```python
from build123d import *

# Parameters (mm, degrees)
SKETCH1_W                           = 558.8
SKETCH1_H                           = 50.8
BOSS_EXTRUDE1_DEPTH                 = 12.7
SKETCH2_W                           = 19.05
SKETCH2_H                           = 44.45
CUT_EXTRUDE1_DEPTH                  = 560.521125607
F_1_4_20_TAPPED_HOLE1_D             = 5.1054
F_10_32_TAPPED_HOLE1_D              = 4.0386
F_10_32_TAPPED_HOLE1_DEPTH          = 5.08
F_10_32_TAPPED_HOLE1_TIP            = 1.213317848
F_5_32_0_15625_DIAMETER_HOLE1_D     = 3.96875
F_5_32_0_15625_DIAMETER_HOLE1_DEPTH = 5.08
F_5_32_0_15625_DIAMETER_HOLE1_TIP   = 1.192332791


with BuildPart() as part:
    # Sketch1 → Boss-Extrude1 (new, symmetric)
    with BuildSketch(Plane.XY):
        Rectangle(SKETCH1_W, SKETCH1_H)
    extrude(amount=BOSS_EXTRUDE1_DEPTH, both=True)

    # Sketch2 → Cut-Extrude1 (cut, through all)
    with BuildSketch(Plane(origin=(279.4, 0, 0), x_dir=(0, 0, -1), z_dir=(1, 0, 0))):
        Rectangle(SKETCH2_W, SKETCH2_H)
    extrude(amount=-CUT_EXTRUDE1_DEPTH, mode=Mode.SUBTRACT)

    # 1/4-20 Tapped Hole1 (through all)
    with Locations(Plane.XY.offset(12.7)):
        with Locations((-260.35, 12.7), (-260.35, -12.7), (260.35, 12.7), (260.35, -12.7)):
            Hole(F_1_4_20_TAPPED_HOLE1_D / 2)

    # #10-32 Tapped Hole1
    with Locations(Plane(origin=(0, 0, -12.7), x_dir=(-1, 0, 0), z_dir=(0, 0, -1))):
        with Locations((-190.5, -13.49375), (-114.3, -13.49375), (-38.1, -13.49375), (38.1, -13.49375), (114.3, -13.49375), (190.5, -13.49375)):
            Hole(F_10_32_TAPPED_HOLE1_D / 2, depth=F_10_32_TAPPED_HOLE1_DEPTH)
            with Locations((0, 0, -(F_10_32_TAPPED_HOLE1_DEPTH + F_10_32_TAPPED_HOLE1_TIP / 2))):  # 118° drill point
                Cone(0, F_10_32_TAPPED_HOLE1_D / 2, F_10_32_TAPPED_HOLE1_TIP, mode=Mode.SUBTRACT)

    # 5/32 (0.15625) Diameter Hole1
    with Locations(Plane(origin=(0, 25.4, 0), x_dir=(1, 0, 0), z_dir=(0, 1, 0))):
        with Locations((-34.925, 0), (34.925, 0)):
            Hole(F_5_32_0_15625_DIAMETER_HOLE1_D / 2, depth=F_5_32_0_15625_DIAMETER_HOLE1_DEPTH)
            with Locations((0, 0, -(F_5_32_0_15625_DIAMETER_HOLE1_DEPTH + F_5_32_0_15625_DIAMETER_HOLE1_TIP / 2))):  # 118° drill point
                Cone(0, F_5_32_0_15625_DIAMETER_HOLE1_D / 2, F_5_32_0_15625_DIAMETER_HOLE1_TIP, mode=Mode.SUBTRACT)


solid = part.part
```
Check sheet for the modelled part. Datum: model origin and axes. Units: mm. A direction names the side the tool comes from. Round coordinates to 2 decimals unless told otherwise and drop trailing zeros. Loops run counter-clockwise (first coordinate to the right, second up) from the corner with the lowest first, then second, coordinate; pieces in that order, holes last. Notation, with made-up numbers: (21.5, 54.5) -> (64.5, 54.5) arc R22 ccw to (64.5, 81.5) -> close; hole circle Ø3 at (75, 8). An arc over 180 degrees is marked (long way). Write item = value, one per line. Start each with the question number.
1) Sectioned sample at B-B, the plane y = -4.5. Record the cut outline in (x, z) (3 decimals), plus the area to 3 significant figures.
2) Thickness scan on probe 1 along Y at (x, z) = (260.35, -11.8); probe 2 along X at (y, z) = (-12, 10.75); probe 3 along Z at (x, y) = (-226, -12) (3 decimals). Record the ranges inside material, lowest first.
3) Gauge pin test, flat ends, axial feed: pin 1 Ø2.5 at (x, y) = (114.3, -13.49) entering from -Z (3 decimals); pin 2 Ø4 at (x, y) = (260.35, 12.7) entering from -Z. Record the tip position at first contact, or that the pin passes through.
4) Sectioned sample at A-A, the plane x = 76.5. Record the cut outline in (y, z) (3 decimals).
5) Release check for a two-part mould opening along Y. For faces 3 (the flat face through (4, -22.225, 0)), 4 (the flat face through (-4, -25.4, 0)), 5 (the flat face through (279.4, 0, 10)), 6 (the flat face through (4, 0, 9.525)) record: released by +Y, released by -Y, zero draft, split by the parting line, or undercut.
6) Set-up check for faces 1 (the flat face through (4, 22.225, 0)), 2 (the flat face through (-4, 0, -12.7)): record each of +Z, -Z, +X, -X, +Y, -Y from which the full face is reachable in a straight line by a thin tool's end or side.
Results are:
q1.outline = (-279.4, -12.7) -> (279.4, -12.7) -> (279.4, -9.525) -> (-279.4, -9.525) -> close; (-279.4, 9.525) -> (279.4, 9.525) -> (279.4, 12.7) -> (-279.4, 12.7) -> close
q1.area = 3,550 mm^2
q2.probe_1 = -25.4 to -15.25, -10.15 to 10.15, 15.25 to 25.4
q2.probe_2 = -279.4 to -262.8, -257.9 to 257.9, 262.8 to 279.4
q2.probe_3 = -12.7 to -9.525, 9.525 to 12.7
q3.pin_1 = 9.525
q3.pin_2 = through
q4.outline = (-25.4, -12.7) -> (25.4, -12.7) -> (25.4, 12.7) -> (-25.4, 12.7) -> close; hole (-22.225, -9.525) -> (22.225, -9.525) -> (22.225, 9.525) -> (-22.225, 9.525) -> close
q5.face_3 = undercut
q5.face_4 = released by -Y
q5.face_5 = zero draft
q5.face_6 = undercut
q6.face_1 = +X, -X
q6.face_2 = -Z, +X, -X, +Y, -Y
